Design review of the part shown in the three views and the two pictorial views. Dimensions are in mm from the part's minimum x, y and z. A direction names the side the tool comes from. Give positions to 0.01 mm unless a question says otherwise; leave off trailing zeros. Loops run counter-clockwise (first coordinate to the right, second up) from the corner with the lowest first, then second, coordinate; pieces in that order, holes last. Notation, with made-up numbers: (59, -35.75) -> (104, -35.75) arc R13 cw to (104, -12.75) -> close; hole circle Ø3 at (-21, 78.25). An arc over 180 degrees is marked (long way). Use CSV: the item, a comma, the result in double quotes. Start each with the question number.
Item 1: We need section D-D (y = 14.75). State the section outline as (x, z) points, plus the area to 3 significant figures.
Item 2: Clearance check with flat-ended pins moving along their axes: pin 1 (1.5 mm diameter, centred on y = 4, z = 7, fed in from -X); pin 2 (5 mm diameter, centred on x = 2.5, z = 8, fed in from +Y); pin 3 (4 mm diameter, centred on x = 8.5, z = 7.5, fed in from -Y); pin 4 (1.5 mm diameter, centred on y = 14.5, z = 8, fed in from +X). State where each tip first meets the part, or that it passes through.
Item 3: We need section C-C (z = 11). State the section outline as (x, y) points.
Item 4: Wall thickness on line 1 along Y through (x, z) = (9, 8.65); line 2 along X through (y, z) = (10.5, 8.25); line 3 along Z through (x, y) = (4.5, 4.25): over which ranges is each line inside the solid? List them lowest first. Write a range as from..to.
Item 5: For the marked faces 1 and 2, list the 3-axis set-ups (+Z, -Z, +X, -X, +Y, -Y) from which the entire face can be reached by the end or side of a thin tool; tool diameter is ignored.
Item 6: We need section A-A (y = 9). State the section outline as (x, z) points, plus the area to 3 significant figures.
Item 7: The part is to be moulded in two halves that separate along X. For the marked faces 3, 4, 5 and 6, say which applies: +X half, -X half, draft (parallel to the pull), parting line (faces both ways), or undercut.
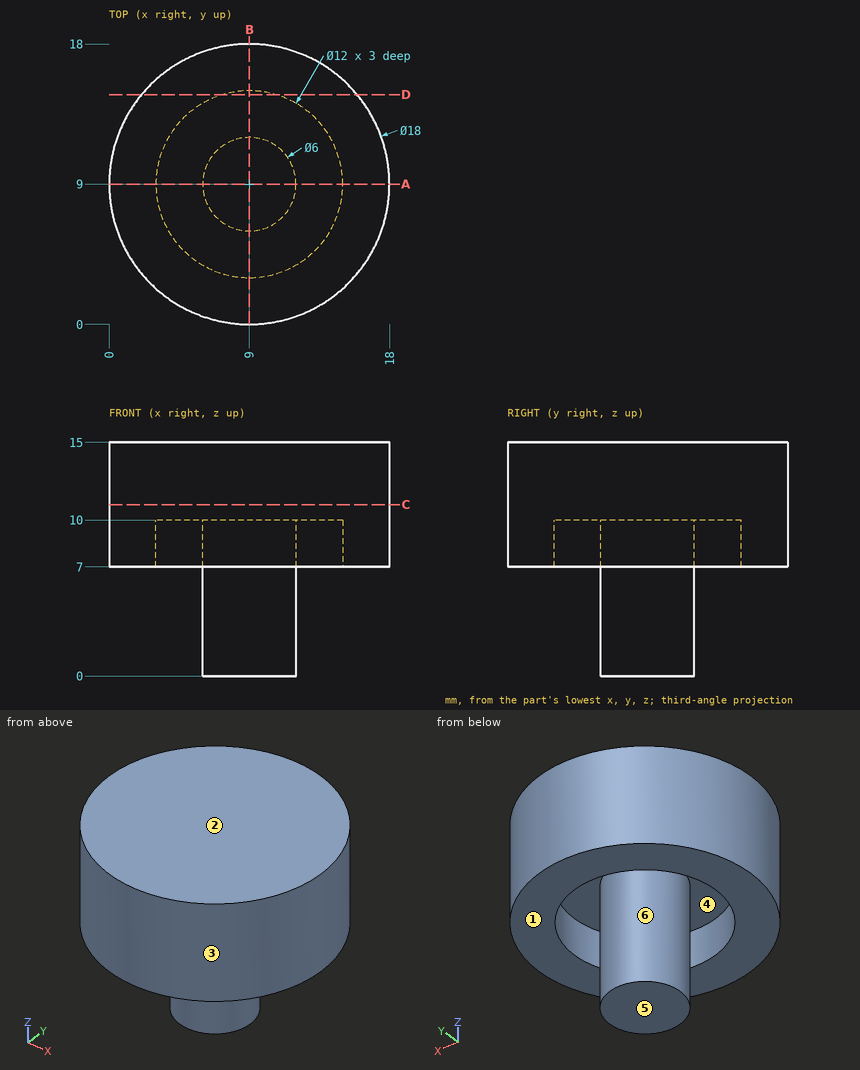
Results found:
1,outline,"(2.08, 7) -> (7.29, 7) -> (7.29, 10) -> (10.71, 10) -> (10.71, 7) -> (15.92, 7) -> (15.92, 15) -> (2.08, 15) -> close"
1,area,"100 mm²"
2,pin 1,"x = 1.07"
2,pin 2,"y = 17.06"
2,pin 3,"y = 0"
2,pin 4,"x = 16.64"
3,outline,"circle Ø18 at (9, 9)"
4,line 1,"0..3, 6..12, 15..18"
4,line 2,"0.13..3.19, 6.4..11.6, 14.81..17.87"
4,line 3,"7..15"
5,face 1,"-Z"
5,face 2,"+Z, +X, -X, +Y, -Y"
6,outline,"(0, 7) -> (3, 7) -> (3, 10) -> (6, 10) -> (6, 0) -> (12, 0) -> (12, 10) -> (15, 10) -> (15, 7) -> (18, 7) -> (18, 15) -> (0, 15) -> close"
6,area,"168 mm²"
7,face 3,"parting line"
7,face 4,"undercut"
7,face 5,"draft"
7,face 6,"undercut"
